Check sheet for the drawn part. Datum: minimum x, y, z corner. Units: mm. Coordinates: 2 decimals unless noted, no trailing zeros. Write each loop counter-clockwise with the first axis right and the second up, starting at its lowest first coordinate (ties: lowest second). Pieces come first, ordered by that corner, then holes. Notation, with made-up numbers: M 0,42.5 L 6,42.5 A31 cw 6,69.5 Z; hole C 68.25,-14.75 d4. An arc over 180 degrees is marked long. Write item = value, one per line. Start each with the question number.
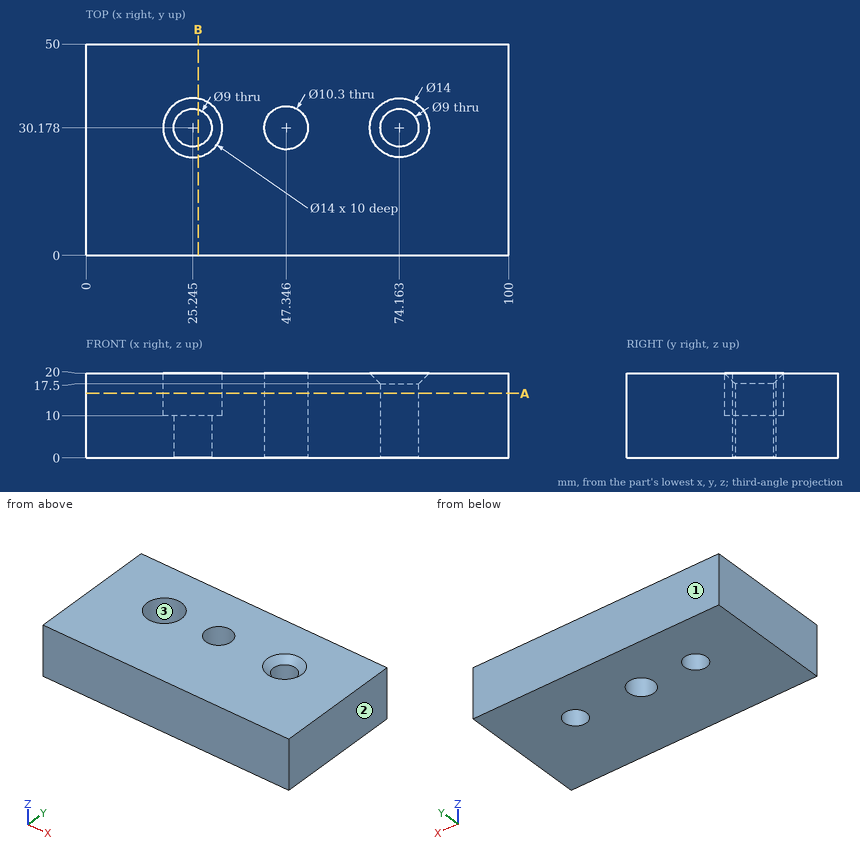
Q1. Draft check along X on the marked faces 1, 2 and 3. Enter one of: pulls with the +X half, pulls with the -X half, needs draft (parallel to the pull), parting line crosses it, or undercut.
Q2. Gauge pin test, flat ends, axial feed: pin 1 (4 mm diameter, centred on x = 26.5, y = 32, fed in from +Z); pin 2 (12.5 mm diameter, centred on x = 25.24, y = 30.18, fed in from -Z). Record the tip position at first contact, or that the pin passes through.
Q3. Cross-section at A-A on z = 15.25. Count the separate pieces of the cut face and the enclosed holes in it, and give its area (3 significant figures).
Q4. Cross-section at B-B on x = 26.5. Enter the section's corners in (y, z) (1 decimal).
Q5. Scan lines: L1, parallel to X at y = 32.5, z = 8.75; L2, parallel to Z at x = 20.5, y = 26.5; L3, parallel to Y at x = 73, z = 4.25 (1 decimal). Record each from-to range of solid material in increasing order.
Values found:
q1.face_1 = needs draft
q1.face_2 = pulls with the +X half
q1.face_3 = undercut
q2.pin_1 = through
q2.pin_2 = 0
q3.separate_pieces = 1
q3.enclosed_holes = 3
q3.area = 4,700 mm²
q4.outline = M 0,0 L 25.9,0 L 25.9,10 L 23.3,10 L 23.3,20 L 0,20 Z; M 34.5,0 L 50,0 L 50,20 L 37.1,20 L 37.1,10 L 34.5,10 Z
q5.L1 = 0 to 21.39, 29.1 to 42.75, 51.94 to 70.31, 78.02 to 100
q5.L2 = 0 to 10
q5.L3 = 0 to 25.8, 34.5 to 50
